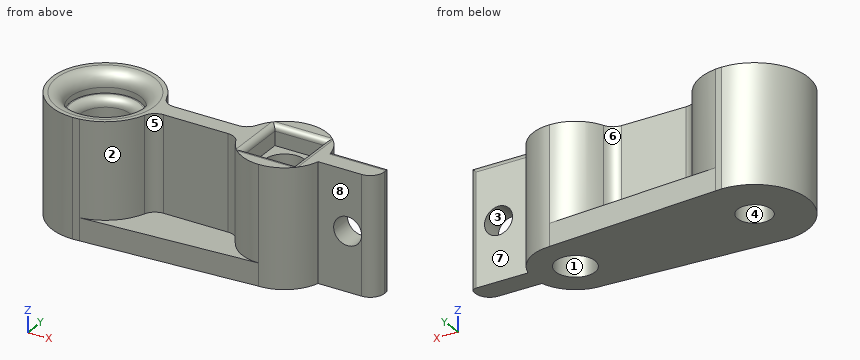
from build123d import *

# Parameters (mm, degrees)
F1_DEPTH       = 21
F1_DEPTH_BACK  = 21
F3_DEPTH       = 34
F4_R           = 6
F4_R_2         = 7
F5_DEPTH       = 42
F6_R           = 9
F6_R_2         = 6
F7_DEPTH       = 22
F8_W           = 18
F8_H           = 18
F8_R           = 7
F9_DEPTH       = 7
F10_R          = 12.5
F11_DEPTH      = 7
F12_R          = 5
F13_DEPTH      = 8
F13_DEPTH_BACK = 8
F14_R          = 4.99999
F15_T1_DEPTH   = 18
F15_T3_DEPTH   = 18
F15_T5_DEPTH   = 52
F15_T10_DEPTH  = 30.5431677052
F15_S11_R      = 15
F15_T12_DEPTH  = 17
F15_T17_DEPTH  = 23
F15_T21_DEPTH  = 23
F15_T28_DEPTH  = 23
F15_T32_DEPTH  = 23
F15_T39_DEPTH  = 23
F15_T43_DEPTH  = 23
F15_T50_DEPTH  = 23
F15_T54_DEPTH  = 23
F16_R          = 2.99999


# Not quite as in the source:
# - a fillet or chamfer that OpenCascade refuses, or shapes differently, is made with other operations: its cross-section is extruded or revolved along the edge and cut away or added
# - a fillet or chamfer is up to 0.001 mm smaller than in the source, because OpenCascade refuses the exact size


with BuildPart() as f1:
    # F0 (on Top) → F1 (new body, two sides)
    with BuildSketch(Plane.XY) as f1_sk:
        with BuildLine():
            Line((4.0776433051, 15), (-57.5565979401, 18.8521400778))
            Line((-57.5565979401, 18.8521400778), (-59.9223566949, 19))
            ThreePointArc((-59.9223566949, 19), (-78.9223566949, 0), (-59.9223566949, -19))
            Line((-59.9223566949, -19), (-57.5565979401, -18.8521400778))
            Line((-57.5565979401, -18.8521400778), (4.0776433051, -15))
            ThreePointArc((4.0776433051, -15), (13.1605943674, -11.9373363863), (18.5344755999, -4))
            ThreePointArc((18.5344755999, -4), (19.0776433051, 0), (18.5344755999, 4))
            ThreePointArc((18.5344755999, 4), (13.1605943674, 11.9373363863), (4.0776433051, 15))
        make_face()
        with BuildLine():
            Line((39.0776433051, 4), (18.5344755999, 4))
            ThreePointArc((18.5344755999, 4), (19.0776433051, 0), (18.5344755999, -4))
            Line((18.5344755999, -4), (39.0776433051, -4))
            Line((39.0776433051, -4), (39.0776433051, 4))
        make_face()
    extrude(amount=F1_DEPTH)
    extrude(f1_sk.sketch, amount=-F1_DEPTH_BACK)

    # F2 (on face) → F3 (cut)
    with BuildSketch(Plane.XY.offset(21)):
        with BuildLine():
            Line((-57.5565979401, -18.8521400778), (-59.9223566949, -19))
            ThreePointArc((-59.9223566949, -19), (-58.737169258, -18.9629989912), (-57.5565979401, -18.8521400778))
        make_face()
        with BuildLine():
            ThreePointArc((-41.1606936556, -3), (-46.7157456922, -13.6596275872), (-57.5565979401, -18.8521400778))
            Line((-57.5565979401, -18.8521400778), (4.0776433051, -15))
            ThreePointArc((4.0776433051, -15), (-5.4091896754, -11.6189500386), (-10.6192951516, -3))
            Line((-10.6192951516, -3), (-41.1606936556, -3))
        make_face()
        with BuildLine():
            Line((-59.9223566949, 19), (-57.5565979401, 18.8521400778))
            ThreePointArc((-57.5565979401, 18.8521400778), (-58.737169258, 18.9629989912), (-59.9223566949, 19))
        make_face()
        with BuildLine():
            ThreePointArc((-10.6192951516, 3), (-5.4091896754, 11.6189500386), (4.0776433051, 15))
            Line((4.0776433051, 15), (-57.5565979401, 18.8521400778))
            ThreePointArc((-57.5565979401, 18.8521400778), (-46.7157456922, 13.6596275872), (-41.1606936556, 3))
            Line((-41.1606936556, 3), (-10.6192951516, 3))
        make_face()
    extrude(amount=-F3_DEPTH, mode=Mode.SUBTRACT)

    # F4 (on face) → F5 (cut)
    with BuildSketch(Plane.XY.offset(21)):
        with Locations((-59.9223566949, 0)):
            Circle(F4_R)
        with Locations((4.0776433051, 0)):
            Circle(F4_R_2)
    extrude(amount=-F5_DEPTH, mode=Mode.SUBTRACT)

    # F6 (on face) → F7 (cut)
    with BuildSketch(Plane.XY.offset(21)):
        with Locations((-59.9223566949, 0)):
            Circle(F6_R)
        with Locations((-59.9223566949, 0)):
            Circle(F6_R_2, mode=Mode.SUBTRACT)
    extrude(amount=-F7_DEPTH, mode=Mode.SUBTRACT)

    # F8 (on face) → F9 (cut)
    with BuildSketch(Plane.XY.offset(21)):
        with Locations((4.0776433051, 0)):
            Rectangle(F8_W, F8_H)
        with Locations((4.0776433051, 0)):
            Circle(F8_R, mode=Mode.SUBTRACT)
    extrude(amount=-F9_DEPTH, mode=Mode.SUBTRACT)

    # F10 (on face) → F11 (cut)
    with BuildSketch(Plane.XY.offset(21)):
        with Locations((-59.9223566949, 0)):
            Circle(F10_R)
    extrude(amount=-F11_DEPTH, mode=Mode.SUBTRACT)

    # F12 (on face) → F13 (cut, two sides)
    with BuildSketch(Plane.XZ.offset(4)) as f13_sk:
        with Locations((29.0776433051, 0)):
            Circle(F12_R)
    extrude(amount=-F13_DEPTH, mode=Mode.SUBTRACT)
    extrude(f13_sk.sketch, amount=F13_DEPTH_BACK, mode=Mode.SUBTRACT)

    # F14 (radius 5 in the source; OpenCascade refuses exactly that, so slightly less here)
    f14_edges = [f1.edges().sort_by_distance(p)[0] for p in [
        (-41.160694, -3, 4),
        (-10.619295, -3, 4),
        (-10.619295, 3, 4),
        (-41.160694, 3, 4),
        (-72.422357, 0, 21),
        (39.077643, -4, 0),
    ]]
    fillet(f14_edges, radius=F14_R)

    # F15: fillet of radius 2 on 6 edges, made by hand

    # F15_s2 → F15_t1 (cut)
    with BuildSketch(Plane.XZ.offset(-9)):
        with BuildLine():
            ThreePointArc((-6.9223566949, 21), (-5.5081431326, 20.4142135624), (-4.9223566949, 19))
            Line((-4.9223566949, 19), (-4.9223566949, 21))
            Line((-4.9223566949, 21), (-6.9223566949, 21))
        make_face()
        with BuildLine():
            ThreePointArc((15.0776433051, 21), (13.6634297427, 20.4142135624), (13.0776433051, 19))
            Line((13.0776433051, 19), (13.0776433051, 21))
            Line((13.0776433051, 21), (15.0776433051, 21))
        make_face()
    extrude(amount=F15_T1_DEPTH, mode=Mode.SUBTRACT)

    # F15_s4 → F15_t3 (cut)
    with BuildSketch(Plane.YZ.offset(-4.9223566949)):
        with BuildLine():
            ThreePointArc((11, 21), (9.5857864376, 20.4142135624), (9, 19))
            Line((9, 19), (9, 21))
            Line((9, 21), (11, 21))
        make_face()
        with BuildLine():
            ThreePointArc((-11, 21), (-9.5857864376, 20.4142135624), (-9, 19))
            Line((-9, 19), (-9, 21))
            Line((-9, 21), (-11, 21))
        make_face()
    extrude(amount=F15_T3_DEPTH, mode=Mode.SUBTRACT)

    # F15_s6 → F15_t5 (cut)
    with BuildSketch(Plane.XY.offset(-26)):
        with BuildLine():
            ThreePointArc((37.0776433051, 4), (38.4918568674, 3.4142135624), (39.0776433051, 2))
            Line((39.0776433051, 2), (39.0776433051, 4))
            Line((39.0776433051, 4), (37.0776433051, 4))
        make_face()
    extrude(amount=F15_T5_DEPTH, mode=Mode.SUBTRACT)


with BuildPart() as f15_tool8:
    # F15_s9 → F15_t10 (new body)
    with BuildSketch(Plane.YZ.offset(44.0776433051)):
        with BuildLine():
            ThreePointArc((2, 21), (3.4142135624, 20.4142135624), (4, 19))
            Line((4, 19), (4, 21))
            Line((4, 21), (2, 21))
        make_face()
    extrude(amount=-F15_T10_DEPTH)

    # F15_s11 → F15_t12 (cut, symmetric)
    with BuildSketch(Plane.XY.offset(20)):
        with Locations((4.0776433051, 0)):
            Circle(F15_S11_R)
    extrude(amount=F15_T12_DEPTH, both=True, mode=Mode.SUBTRACT)


with BuildPart() as f1_1:
    add(f1.part)

    # F15_t7: cut F15_tool8
    add(f15_tool8.part, mode=Mode.SUBTRACT)


with BuildPart() as f15_tool15:
    # F15_s16 → F15_t17 (new body)
    with BuildSketch(Plane.XZ.offset(-14)):
        with BuildLine():
            ThreePointArc((-6.9223566949, 21), (-5.5081431326, 20.4142135624), (-4.9223566949, 19))
            Line((-4.9223566949, 19), (-4.9223566949, 21))
            Line((-4.9223566949, 21), (-6.9223566949, 21))
        make_face()
    extrude(amount=F15_T17_DEPTH)

    split(bisect_by=Plane.XZ.offset(-9), keep=Keep.BOTTOM)


with BuildPart() as f15_tool19:
    # F15_s20 → F15_t21 (new body)
    with BuildSketch(Plane.YZ.offset(13.0776433051)):
        with BuildLine():
            ThreePointArc((11, 21), (9.5857864376, 20.4142135624), (9, 19))
            Line((9, 19), (9, 21))
            Line((9, 21), (11, 21))
        make_face()
    extrude(amount=-F15_T21_DEPTH)

    split(bisect_by=Plane.YZ.offset(-4.9223566949), keep=Keep.BOTTOM)


with BuildPart() as f15_tool15_1:
    add(f15_tool15.part)

    # F15_t23: intersect F15_tool19
    add(f15_tool19.part, mode=Mode.INTERSECT)


with BuildPart() as f1_2:
    add(f1_1.part)

    # F15_t13: cut F15_tool15
    add(f15_tool15_1.part, mode=Mode.SUBTRACT)


with BuildPart() as f15_tool26:
    # F15_s27 → F15_t28 (new body)
    with BuildSketch(Plane.YZ.offset(-9.9223566949)):
        with BuildLine():
            ThreePointArc((-11, 21), (-9.5857864376, 20.4142135624), (-9, 19))
            Line((-9, 19), (-9, 21))
            Line((-9, 21), (-11, 21))
        make_face()
    extrude(amount=F15_T28_DEPTH)

    split(bisect_by=Plane.YZ.offset(-4.9223566949), keep=Keep.BOTTOM)


with BuildPart() as f15_tool30:
    # F15_s31 → F15_t32 (new body)
    with BuildSketch(Plane.XZ.offset(-9)):
        with BuildLine():
            ThreePointArc((-6.9223566949, 21), (-5.5081431326, 20.4142135624), (-4.9223566949, 19))
            Line((-4.9223566949, 19), (-4.9223566949, 21))
            Line((-4.9223566949, 21), (-6.9223566949, 21))
        make_face()
    extrude(amount=F15_T32_DEPTH)

    split(bisect_by=Plane.XZ.offset(9), keep=Keep.TOP)


with BuildPart() as f15_tool26_1:
    add(f15_tool26.part)

    # F15_t34: intersect F15_tool30
    add(f15_tool30.part, mode=Mode.INTERSECT)


with BuildPart() as f1_3:
    add(f1_2.part)

    # F15_t24: cut F15_tool26
    add(f15_tool26_1.part, mode=Mode.SUBTRACT)


with BuildPart() as f15_tool37:
    # F15_s38 → F15_t39 (new body)
    with BuildSketch(Plane.XZ.offset(9)):
        with BuildLine():
            ThreePointArc((15.0776433051, 21), (13.6634297427, 20.4142135624), (13.0776433051, 19))
            Line((13.0776433051, 19), (13.0776433051, 21))
            Line((13.0776433051, 21), (15.0776433051, 21))
        make_face()
    extrude(amount=-F15_T39_DEPTH)

    split(bisect_by=Plane.XZ.offset(-9), keep=Keep.BOTTOM)


with BuildPart() as f15_tool41:
    # F15_s42 → F15_t43 (new body)
    with BuildSketch(Plane.YZ.offset(18.0776433051)):
        with BuildLine():
            ThreePointArc((11, 21), (9.5857864376, 20.4142135624), (9, 19))
            Line((9, 19), (9, 21))
            Line((9, 21), (11, 21))
        make_face()
    extrude(amount=-F15_T43_DEPTH)

    split(bisect_by=Plane.YZ.offset(13.0776433051), keep=Keep.TOP)


with BuildPart() as f15_tool37_1:
    add(f15_tool37.part)

    # F15_t45: intersect F15_tool41
    add(f15_tool41.part, mode=Mode.INTERSECT)


with BuildPart() as f1_4:
    add(f1_3.part)

    # F15_t35: cut F15_tool37
    add(f15_tool37_1.part, mode=Mode.SUBTRACT)


with BuildPart() as f15_tool48:
    # F15_s49 → F15_t50 (new body)
    with BuildSketch(Plane.YZ.offset(-4.9223566949)):
        with BuildLine():
            ThreePointArc((-11, 21), (-9.5857864376, 20.4142135624), (-9, 19))
            Line((-9, 19), (-9, 21))
            Line((-9, 21), (-11, 21))
        make_face()
    extrude(amount=F15_T50_DEPTH)

    split(bisect_by=Plane.YZ.offset(13.0776433051), keep=Keep.TOP)


with BuildPart() as f15_tool52:
    # F15_s53 → F15_t54 (new body)
    with BuildSketch(Plane.XZ.offset(14)):
        with BuildLine():
            ThreePointArc((15.0776433051, 21), (13.6634297427, 20.4142135624), (13.0776433051, 19))
            Line((13.0776433051, 19), (13.0776433051, 21))
            Line((13.0776433051, 21), (15.0776433051, 21))
        make_face()
    extrude(amount=-F15_T54_DEPTH)

    split(bisect_by=Plane.XZ.offset(9), keep=Keep.TOP)


with BuildPart() as f15_tool48_1:
    add(f15_tool48.part)

    # F15_t56: intersect F15_tool52
    add(f15_tool52.part, mode=Mode.INTERSECT)


with BuildPart() as f1_5:
    add(f1_4.part)

    # F15_t46: cut F15_tool48
    add(f15_tool48_1.part, mode=Mode.SUBTRACT)

    # F16 (radius 3 in the source; OpenCascade refuses exactly that, so slightly less here)
    f16_edges = [f1_5.edges().sort_by_distance(p)[0] for p in [
        (-68.922357, 0, 14),
        (-65.922357, 0, -1),
    ]]
    fillet(f16_edges, radius=F16_R)


solid = f1_5.part
Check sheet for the modelled part. Datum: model origin and axes. Units: mm. Face numbers are marked on the shaded views. A direction names the side the tool comes from. Coordinates: 2 decimals unless noted, no trailing zeros. Write each loop counter-clockwise with the first axis right and the second up, starting at its lowest first coordinate (ties: lowest second). Pieces come first, ordered by that corner, then holes. Notation, with made-up numbers: M 9,50.25 L 51,50.25 A22 ccw 51,75.25 Z; hole C -9.75,-27 d10. An arc over 180 degrees is marked long. Answer as CSV lines item,"result".
Q1. Cross-section at A-A (z = -11). Record the boundary of the cut face in (x, y).
Check result:
outline,"M -59.92,-19 L -57.56,-18.85 A19 ccw -42.01,-6.33 A5 cw -37.29,-3 L -14.25,-3 A5 cw -9.67,-6 A15 ccw 18.53,-4 L 34.08,-4 A5 ccw 39.08,1 L 39.08,2 A2 ccw 37.08,4 L 18.53,4 A15 ccw -9.67,6 A5 cw -14.25,3 L -37.29,3 A5 cw -42.01,6.33 A19 ccw -57.56,18.85 L -59.92,19 A19 ccw Z; hole C -59.92,0 d12; hole C 4.08,0 d14"
Q2. Mould release check, pull along Y, two halves, no side actions. Record for the marked faces 1, 2 and 3: released by +Y, released by -Y, zero draft, split by the parting line, or undercut.
Check result:
face 1,"undercut"
face 2,"released by -Y"
face 3,"zero draft"
Q3. Go/stop test with flat-tipped pins: pin 1 (2.5 mm diameter, centred on x = 8.5, z = 16.5, fed in from -Y); pin 2 (15 mm diameter, centred on x = 32.5, z = -3, fed in from +Y); pin 3 (1.5 mm diameter, centred on y = 14.5, z = -3.5, fed in from +X); pin 4 (15 mm diameter, centred on x = -59.92, y = 0, fed in from -Z). Record where each tip stops, or that it passes through.
Check result:
pin 1,"y = -14.66"
pin 2,"y = 4"
pin 3,"x = 10.07"
pin 4,"z = -21"
Q4. Set-up check for the marked faces 4, 5, 6, 7 and 8: record each of +Z, -Z, +X, -X, +Y, -Y from which the full face is reachable in a straight line by a thin tool's end or side.
Check result:
face 4,"+Z, -Z"
face 5,"+Z, -Y"
face 6,"+Z, +Y"
face 7,"+Z, -Z, +X, +Y"
face 8,"+Z, -Z, +X, -Y"
Q5. Cross-section at B-B (x = -22). Record the boundary of the cut face in (y, z), then the cut area to 3 significant figures.
Check result:
outline,"M -16.63,-21 L 16.63,-21 L 16.63,-13 L 3,-13 L 3,21 L -3,21 L -3,-13 L -16.63,-13 Z"
area,"470 mm^2"
Q6. Material ranges on probe 1 along X at (y, z) = (-1.5, -19); probe 2 along Y at (x, z) = (-60, -18.5); probe 3 along X at (y, z) = (6, 1), recorded low to high. Write a range as from..to.
Check result:
probe 1,"-78.86..-65.73, -54.11..-2.76, 10.92..38.41"
probe 2,"-19..-6, 6..19"
probe 3,"-77.95..-66.63, -53.21..-41.88, -9.67..0.47, 7.68..17.83"
